Could you check a few things on this drawing? It's one solid part, dimensions in mm from its lowest x, y, z. A direction names the side the tool comes from. Give positions to 0.01 mm unless a question says otherwise; leave off trailing zeros. Loops run counter-clockwise (first coordinate to the right, second up) from the corner with the lowest first, then second, coordinate; pieces in that order, holes last.
Q1. For the marked faces 1, 2 and 3, which set-ups out of +Z, -Z, +X, -X, +Y, -Y let a thin tool reach every point of the face, with its end or its side?
Q2. Thinking about a two-plate mould opening in Z: for the marked faces 4, 5, 6 and 7, which applies, pulls with the +Z half, pulls with the -Z half, needs draft (parallel to the pull), parting line crosses it, or undercut?
Q3. I need wall thicknesses on probe 1 along Z at (x, y) = (14.5, 9.5); probe 2 along X at (y, z) = (5.5, 4.5); probe 3 along Y at (x, z) = (17.75, 8). Which ranges of each line are inside material? Lowest first, please.
Q4. I'm going to push flat-ended pins straight in: P1, Ø1.2, axis at x = 7.5, z = 2, coming from the -Y side; P2, Ø4.5, axis at x = 7.5, y = 1.5, coming from the +Z side; P3, Ø6, axis at y = 11.5, z = 14.5, coming from the +X side; P4, Ø6, axis at x = 18.5, z = 14, coming from the -Y side. Where does each tip first touch, or does it pass through?
Q5. Suppose I cut it at A-A (z = 8.45). List the corners of the cut face in (x, y) for me.
Q6. Suppose I cut it at D-D (y = 5.25). List the corners of the cut face in (x, z) for me, and give its area (3 significant figures).
Q7. Suppose I cut it at B-B (x = 3.25). List the corners of the cut face in (y, z) for me.
Q8. Suppose I cut it at C-C (x = 16.5). List the corners of the cut face in (y, z) for me.
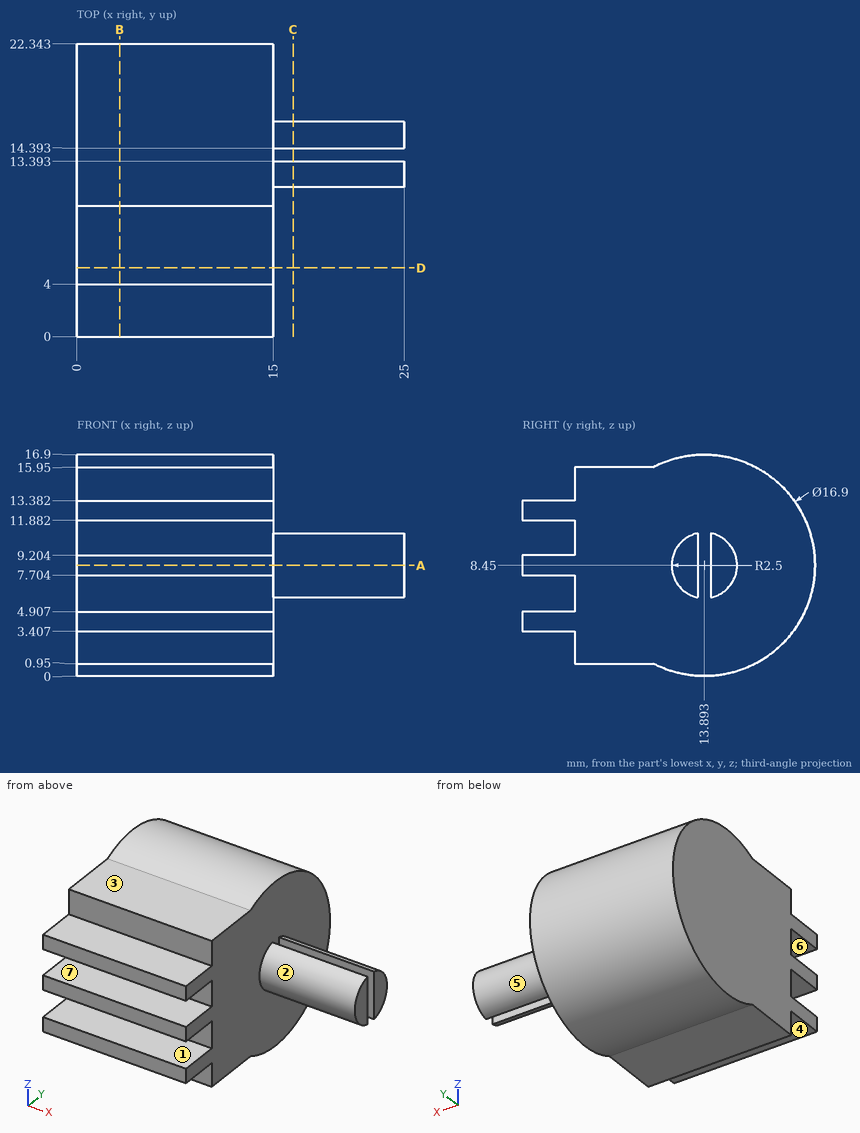
Solutions:
1. face 1: +X, -X, -Y
1. face 2: +X, -Y
1. face 3: +Z, +X, -X, -Y
2. face 4: pulls with the -Z half
2. face 5: parting line crosses it
2. face 6: undercut
2. face 7: undercut
3. probe 1: z = 0.95 to 15.95
3. probe 2: x = 0 to 15
3. probe 3: y = 11.43 to 13.39, 14.39 to 16.35
4. P1: stops at y = 4
4. P2: stops at z = 13.38
4. P3: stops at x = 15
4. P4: passes through
5. outline: (0, 0) - (15, 0) - (15, 11.39) - (25, 11.39) - (25, 13.39) - (15, 13.39) - (15, 14.39) - (25, 14.39) - (25, 16.39) - (15, 16.39) - (15, 22.34) - (0, 22.34) - close
6. outline: (0, 0.95) - (15, 0.95) - (15, 15.95) - (0, 15.95) - close
6. area: 225 mm2
7. outline: (0, 3.41) - (4, 3.41) - (4, 0.95) - (10, 0.95) arc R8.45 ccw (long way) to (10, 15.95) - (4, 15.95) - (4, 13.38) - (0, 13.38) - (0, 11.88) - (4, 11.88) - (4, 9.2) - (0, 9.2) - (0, 7.7) - (4, 7.7) - (4, 4.91) - (0, 4.91) - close
8. outline: (13.39, 6) - (13.39, 10.9) arc R2.5 ccw to start; (14.39, 6) arc R2.5 ccw to (14.39, 10.9) - close
